Work out the finished part from the listing and answer in its coordinate system (mm). Round coordinates to 2 decimals unless told otherwise and drop trailing zeros. Loops run counter-clockwise (first coordinate to the right, second up) from the corner with the lowest first, then second, coordinate; pieces in that order, holes last. Notation, with made-up numbers: (-0.5, 70.5) - (46.5, 70.5) arc R23 ccw to (46.5, 85.5) - close; hole circle Ø7 at (64, 21). An arc over 180 degrees is marked (long way). Use CSV: the item, a comma, the result in double quotes. Start each with the question number.
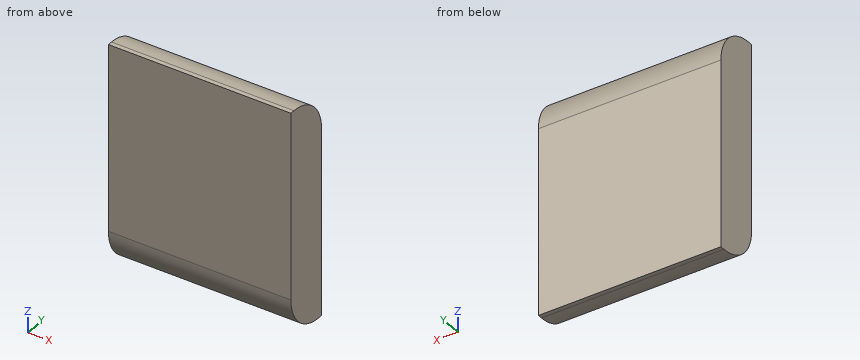
from build123d import *

# Parameters (mm, degrees)
F0_W     = 10.16
F0_H     = 12.7
F1_DEPTH = 2.54
F2_R     = 2.286
F3_R     = 2.286


with BuildPart() as f1:
    # F0 (on Front) → F1 (new body)
    with BuildSketch(Plane.XZ):
        Rectangle(F0_W, F0_H)
    extrude(amount=F1_DEPTH)

    # F2
    f2_edges = [f1.edges().sort_by_distance(p)[0] for p in [
        (0, -2.54, -6.35),
    ]]
    fillet(f2_edges, radius=F2_R)

    # F3
    f3_edges = [f1.edges().sort_by_distance(p)[0] for p in [
        (0, 0, 6.35),
    ]]
    fillet(f3_edges, radius=F3_R)


solid = f1.part
Item 1: A cutting plane is placed at A-A (x = -1.75). Determine the outline of the cut face in (y, z).
Item 2: A cutting plane is placed at B-B (z = -5). Determine the outline of the cut face in (x, y), plus the area to 3 significant figures.
Item 3: Find the intervals of material crossed by probe 1 along Z at (x, y) = (-4, -0.9); probe 2 along Y at (x, z) = (3, 5); probe 3 along Z at (x, y) = (-1.5, -0.4), in increasing order. Write a range as [from, to].
Item 4: This flat-tipped pin is pushed along its axis until it touches: pin 1 Ø1.5 at (x, y) = (1.5, -1.5) entering from -Z. Where does it stop, or does it pass through?
Item 5: A cutting plane is placed at C-C (y = -1). Determine the outline of the cut face in (x, z), plus the area to 3 significant figures.
Result sheet:
1,outline,"(-2.54, -4.06) arc R2.29 ccw to (-0.25, -6.35) - (0, -6.35) - (0, 4.06) arc R2.29 ccw to (-2.29, 6.35) - (-2.54, 6.35) - close"
2,outline,"(-5.08, -2.34) - (5.08, -2.34) - (5.08, 0) - (-5.08, 0) - close"
2,area,"23.8 mm^2"
3,probe 1,"[-6.26, 5.88]"
3,probe 2,"[-2.54, -0.2]"
3,probe 3,"[-6.35, 5.36]"
4,pin 1,"z = -6.3"
5,outline,"(-5.08, -6.22) - (5.08, -6.22) - (5.08, 5.95) - (-5.08, 5.95) - close"
5,area,"124 mm^2"
